```python
from build123d import *

# Parameters (mm, degrees)
EXTRUDE_1_DEPTH     = 6
SKETCH_8_W          = 30
SKETCH_8_H          = 4.5
EXTRUDE_4_DEPTH     = 4.5
CHAMFER_1_SIZE      = 2
CHAMFER_2_SIZE      = 2
CUT_EXTRUDE_2_REACH = 26.75
SKETCH_8_5_R        = 7.5
SKETCH_13_W         = 30
SKETCH_13_H         = 6
EXTRUDE_5_DEPTH     = 4.5


# Read off the part's stored shape, not the designer's step: the mirror step
with BuildPart() as part:
    # Sketch 1 → Extrude 1 (new body)
    with BuildSketch(Plane.XY):
        Polygon((-13, 18.75), (-15, 16.75), (-15, -18.75), (15, -18.75), (15, 16.75), (13, 18.75), align=None)
    extrude(amount=EXTRUDE_1_DEPTH)

    # Sketch 8 → Extrude 4 (add)
    with BuildSketch(Plane.XY.offset(6)):
        with Locations((0, -16.5)):
            Rectangle(SKETCH_8_W, SKETCH_8_H)
    extrude(amount=EXTRUDE_4_DEPTH)

    # Chamfer 1
    chamfer_1_edges = [part.edges().sort_by_distance(p)[0] for p in [
        (-15, -16.5, 10.5),
    ]]
    chamfer(chamfer_1_edges, length=CHAMFER_1_SIZE)

    # Chamfer 2
    chamfer_2_edges = [part.edges().sort_by_distance(p)[0] for p in [
        (15, -16.5, 10.5),
    ]]
    chamfer(chamfer_2_edges, length=CHAMFER_2_SIZE)

    # Sketch 8_5 → Cut-Extrude 2 (cut, up to next)
    with BuildSketch(Plane.XY.offset(6), mode=Mode.PRIVATE) as cut_extrude_2_sk1:
        with Locations((0, 6.75)):
            Circle(SKETCH_8_5_R)
    cut_extrude_2_tool1 = extrude(cut_extrude_2_sk1.sketch, amount=-CUT_EXTRUDE_2_REACH, mode=Mode.PRIVATE) & part.part
    add(cut_extrude_2_tool1.solids().sort_by_distance((0, 6.75, 6))[0], mode=Mode.SUBTRACT)

    # Sketch 13 → Extrude 5 (add)
    with BuildSketch(Plane(origin=(0, 0, 0), x_dir=(-1, 0, 0), z_dir=(0, 0, -1))):
        with Locations((0, -15.75)):
            Rectangle(SKETCH_13_W, SKETCH_13_H)
    extrude(amount=EXTRUDE_5_DEPTH)

    # Mirror 4: part across plane


with BuildPart() as part_1:
    add(part.part)
    add(part.part.mirror(Plane(origin=(0, 0, -4.5), x_dir=(1, 0, 0), z_dir=(0, 0, -1))))


solid = part_1.part
```
Verification items for the finished model (mm, model axes). A direction names the side the tool comes from. Give positions to 0.01 mm unless a question says otherwise; leave off trailing zeros. Order: outer loops, then holes, each group sorted by start corner. A loop starts at its lowest first (then second) coordinate and runs counter-clockwise, first axis right, second up. Notation, with made-up numbers: (30.25, 35.25) -> (80.25, 35.25) arc R9 cw to (80.25, 46.25) -> close; hole circle Ø3 at (-3, 4). An arc over 180 degrees is marked (long way). One line per item, written item: value.
(1) Tool access check on faces 4 (the face through (0, -1, 6)), 5 (the face through (0, 18.75, -12)), 6 (the face through (-4, 0, -9)), 7 (the face through (14, -16.5, 9.5)), 8 (the face through (0, -1, -15)). Record the directions out of +Z, -Z, +X, -X, +Y, -Y that give a thin tool (end or side, any length) a straight path to the whole face; none if there is none.
Final values:
face 4: +Z, +X, -X, +Y
face 5: +Z, -Z, +X, -X, +Y
face 6: +X, -X, +Y
face 7: +Z, +X, +Y, -Y
face 8: -Z, +X, -X, +Y
(2) Scan lines: line 1 along Z through (x, y) = (-6.75, 16); line 2 along Y through (x, z) = (0, -11.2); line 3 along Z through (x, y) = (4.75, -13). Record each from-to range of solid material in increasing order. Write a range as [from, to].
Final values:
line 1: [-15, -9], [0, 6]
line 2: [-18.75, -0.75], [14.25, 18.75]
line 3: [-15, 6]
(3) Sectioned sample at B-B on z = 0.5. Record the cut outline in (x, y), then the cut area to 3 significant figures.
Final values:
outline: (-15, -18.75) -> (15, -18.75) -> (15, 16.75) -> (13, 18.75) -> (-13, 18.75) -> (-15, 16.75) -> close; hole circle Ø15 at (0, 6.75)
area: 944 mm^2
(4) Gauge pin test, flat ends, axial feed: pin 1 (1.3 mm diameter, centred on x = -2, z = 8.5, fed in from +Y); pin 2 (12 mm diameter, centred on x = 0, y = 14.5, fed in from +Z); pin 3 (4.5 mm diameter, centred on x = -2, z = -3, fed in from +Y). Record the tip position at first contact, or that the pin passes through.
Final values:
pin 1: y = -14.25
pin 2: z = 6
pin 3: y = -12.75
(5) Draft check along Z on faces 1 (the face through (-4, 0, 0)), 2 (the face through (0, -16, -19.5)), 3 (the face through (0, -16, 10.5)). Enter one of: pulls with the +Z half, pulls with the -Z half, needs draft (parallel to the pull), parting line crosses it, or undercut.
Final values:
face 1: undercut
face 2: pulls with the -Z half
face 3: pulls with the +Z half
(6) Sectioned sample at A-A on x = 6. Record the cut outline in (y, z), then the cut area to 4 significant figures.
Final values:
outline: (-18.75, -19.5) -> (-14.25, -19.5) -> (-14.25, -15) -> (2.25, -15) -> (2.25, -9) -> (-12.75, -9) -> (-12.75, 0) -> (2.25, 0) -> (2.25, 6) -> (-14.25, 6) -> (-14.25, 10.5) -> (-18.75, 10.5) -> close; (11.25, -15) -> (18.75, -15) -> (18.75, -9) -> (11.25, -9) -> close; (11.25, 0) -> (18.75, 0) -> (18.75, 6) -> (11.25, 6) -> close
area: 436.5 mm^2
(7) Sectioned sample at D-D on y = -7. Record the cut outline in (x, z), then the cut area to 3 significant figures.
Final values:
outline: (-15, -15) -> (15, -15) -> (15, -9) -> (-15, -9) -> close; (-15, 0) -> (15, 0) -> (15, 6) -> (-15, 6) -> close
area: 360 mm^2
(8) Sectioned sample at C-C on y = 6.75. Record the cut outline in (x, z), then the cut area to 3 significant figures.
Final values:
outline: (-15, -15) -> (-7.5, -15) -> (-7.5, -9) -> (-15, -9) -> close; (-15, 0) -> (-7.5, 0) -> (-7.5, 6) -> (-15, 6) -> close; (7.5, -15) -> (15, -15) -> (15, -9) -> (7.5, -9) -> close; (7.5, 0) -> (15, 0) -> (15, 6) -> (7.5, 6) -> close
area: 180 mm^2
